Read the model definition and answer for the solid it produces. Units are mm, in the model's axes. A direction names the side the tool comes from. Round coordinates to 2 decimals unless told otherwise and drop trailing zeros. Write each loop counter-clockwise with the first axis right and the second up, starting at its lowest first coordinate (ties: lowest second). Pieces come first, ordered by that corner, then holes. Notation, with made-up numbers: (83, -13.75) -> (88, -13.75) arc R22 cw to (88, 5.25) -> close; hole circle Ø4 at (8, 54). An arc over 180 degrees is marked (long way). Return JSON: item names as keys, results as strings. Group by question number.
(1) The mould has two halves that part along Y. Classify faces 3 (the flat face through (15, 0, 2)), 4 (the cylindrical face through (-13.04, -26.41, 2.41)), 5 (the flat face through (5, 9, 2)): released by +Y, released by -Y, zero draft, split by the parting line, or undercut.
(2) For faces 1 (the flat face through (5, -8, 2)), 2 (the flat face through (0, -32, 2)), determine the directions among +Z, -Z, +X, -X, +Y, -Y from which every point of the face is accessible in a straight line to the end or side of a thin tool.
(3) Straight lines are drawn through the part: line 1 (X direction, y = 17, z = 1.1); line 2 (X direction, y = -6, z = 0.65); line 3 (Y direction, x = 7, z = 3.8). For each, find the intervals that lie inside material, in ascending order.
(4) Given pin 1 (9.5 mm diameter, centred on x = 0, y = -16, fed in from +Z); pin 2 (1 mm diameter, centred on x = 3.5, z = 1, fed in from +Y); pin 3 (1.5 mm diameter, centred on y = 27.5, z = 4, fed in from -X), each flat-ended and moving along its own axis, determine where each tip first touches the part or whether it passes through.
(5) A cutting plane is placed at B-B on y = -16. Give the vertices of the cut face in (x, z).
(6) A cutting plane is placed at C-C on x = 12. Give the vertices of the cut face in (y, z).
```python
from build123d import *

# Parameters (mm, degrees)
CROQUIS1_W              = 30
CROQUIS1_H              = 68
SALIENTE_EXTRUIR1_DEPTH = 4.7625
REDONDEO1_R             = 15
CROQUIS2_R              = 8
CORTAR_EXTRUIR1_DEPTH   = 10
CROQUIS3_W              = 31.404872341
CROQUIS3_H              = 7.197905048
CORTAR_EXTRUIR2_DEPTH   = 10


with BuildPart() as part:
    # Croquis1 → Saliente-Extruir1 (new body)
    with BuildSketch(Plane.XY):
        Rectangle(CROQUIS1_W, CROQUIS1_H)
        with BuildLine():
            Line((5, 14), (5, -14))
            ThreePointArc((5, -14), (0, -19), (-5, -14))
            Line((-5, -14), (-5, 14))
            ThreePointArc((-5, 14), (0, 19), (5, 14))
        make_face(mode=Mode.SUBTRACT)
    extrude(amount=SALIENTE_EXTRUIR1_DEPTH)

    # Redondeo1
    redondeo1_edges = [part.edges().sort_by_distance(p)[0] for p in [
        (15, -34, 2.38125),
        (-15, -34, 2.38125),
        (-15, 34, 2.38125),
        (15, 34, 2.38125),
    ]]
    fillet(redondeo1_edges, radius=REDONDEO1_R - 0.0001)  # a hair under: the kernel refuses the full size

    # Croquis2 → Cortar-Extruir1 (cut)
    with BuildSketch(Plane.XY.offset(4.7625)):
        with Locations((0, 17)):
            Circle(CROQUIS2_R)
        with Locations((0, 0.5)):
            Circle(CROQUIS2_R)
        with Locations((0, -16)):
            Circle(CROQUIS2_R)
    extrude(amount=-CORTAR_EXTRUIR1_DEPTH, mode=Mode.SUBTRACT)

    # Croquis3 → Cortar-Extruir2 (cut)
    with BuildSketch(Plane.XY.offset(4.7625)):
        with Locations((0.058431815, -35.598952524)):
            Rectangle(CROQUIS3_W, CROQUIS3_H)
    extrude(amount=-CORTAR_EXTRUIR2_DEPTH, mode=Mode.SUBTRACT)


solid = part.part
```
Checks:
{
 "1": {"face 3": "zero draft", "face 4": "released by -Y", "face 5": "undercut"},
 "2": {"face 1": "+Z, -Z", "face 2": "+Z, -Z, +X, -X, -Y"},
 "3": {"line 1": "x = -15 to -8, 8 to 15", "line 2": "x = -15 to -5, 5 to 15", "line 3": "y = -32 to -19.87, -12.13 to -3.37, 4.37 to 13.13, 20.87 to 32.27"},
 "4": {"pin 1": "passes through", "pin 2": "stops at y = 33.7", "pin 3": "stops at x = -12.84"},
 "5": {"outline": "(-15, 0) -> (-8, 0) -> (-8, 4.76) -> (-15, 4.76) -> close; (8, 0) -> (15, 0) -> (15, 4.76) -> (8, 4.76) -> close"},
 "6": {"outline": "(-28, 0) -> (28, 0) -> (28, 4.76) -> (-28, 4.76) -> close"}
}
